from build123d import *

# Parameters (mm, degrees)
ESQUISSE2_W             = 33
ESQUISSE2_H             = 51
ENL_V_MAT_EXTRU_1_DEPTH = 41
ESQUISSE3_W             = 8
ESQUISSE3_H             = 12
ESQUISSE3_W_2           = 12
ESQUISSE3_H_2           = 8
ENL_V_MAT_EXTRU_3_DEPTH = 42
ESQUISSE4_W             = 23.524420498
ESQUISSE4_H             = 14.572913479
ENL_V_MAT_EXTRU_4_DEPTH = 269
ESQUISSE6_R             = 2.08560847
ENL_V_MAT_EXTRU_5_DEPTH = 10


with BuildPart() as part:
    # Esquisse1 → Révolution1 (revolve)
    with BuildSketch(Plane.XY, mode=Mode.PRIVATE) as r_volution1_sk:
        Polygon((0, 0), (-50, 0), (-35, 45), (0, 45), align=None)
    revolve(r_volution1_sk.sketch.rotate(Axis((0, 185.624886126, 0), (0, -1, 0)), 270), axis=Axis((0, 185.624886126, 0), (0, -1, 0)))

    # Esquisse2 → Enlèv. mat.-Extru.1 (cut)
    with BuildSketch(Plane(origin=(0, 45, 0), x_dir=(1, 0, 0), z_dir=(0, 1, 0))):
        Rectangle(ESQUISSE2_W, ESQUISSE2_H)
    extrude(amount=-ENL_V_MAT_EXTRU_1_DEPTH, mode=Mode.SUBTRACT)

    # Esquisse3 → Enlèv. mat.-Extru.3 (cut)
    with BuildSketch(Plane(origin=(0, 45, 0), x_dir=(1, 0, 0), z_dir=(0, 1, 0))):
        with Locations((0, 46)):
            Rectangle(ESQUISSE3_W, ESQUISSE3_H)
        with Locations((46, 0)):
            Rectangle(ESQUISSE3_W_2, ESQUISSE3_H_2)
        with Locations((0, -46)):
            Rectangle(ESQUISSE3_W, ESQUISSE3_H)
        with Locations((-46, 0)):
            Rectangle(ESQUISSE3_W_2, ESQUISSE3_H_2)
    extrude(amount=-ENL_V_MAT_EXTRU_3_DEPTH, mode=Mode.SUBTRACT)

    # Esquisse4 → Enlèv. mat.-Extru.4 (cut)
    with BuildSketch(Plane(origin=(0, 4, 0), x_dir=(1, 0, 0), z_dir=(0, 1, 0))):
        with Locations((-1.026102351, -0.627863405)):
            Rectangle(ESQUISSE4_W, ESQUISSE4_H)
    extrude(amount=-ENL_V_MAT_EXTRU_4_DEPTH, mode=Mode.SUBTRACT)

    # Esquisse6 → Enlèv. mat.-Extru.5 (cut)
    with BuildSketch(Plane(origin=(0, 3, 0), x_dir=(1, 0, 0), z_dir=(0, 1, 0))):
        with Locations(Location((0, 44.460655409, 0), (0, 0, 270))):
            Circle(ESQUISSE6_R)
    extrude(amount=-ENL_V_MAT_EXTRU_5_DEPTH, mode=Mode.SUBTRACT)


solid = part.part
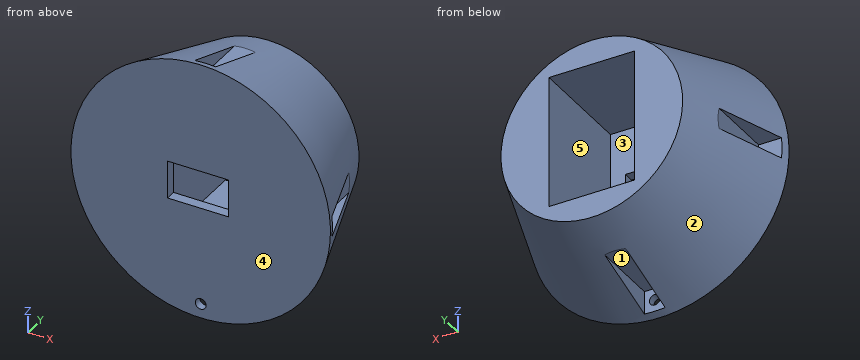
Read the model definition and answer for the solid it produces. Units are mm, in the model's axes. Face numbers are marked on the shaded views. A direction names the side the tool comes from. Give positions to 0.01 mm unless a question says otherwise; leave off trailing zeros. Loops run counter-clockwise (first coordinate to the right, second up) from the corner with the lowest first, then second, coordinate; pieces in that order, holes last. Notation, with made-up numbers: M 22,39.5 L 36,39.5 A19 ccw 36,69.5 Z; hole C -33.5,-34 d6. An arc over 180 degrees is marked long. Write each question's results on one line, items separated by ' | '.
1. Section A-A on z = 0 is taken. Give the vertices of the cut face in (x, y), plus the area to 3 significant figures.
Values:
outline: M -50,0 L -12.79,0 L -12.79,4 L -16.5,4 L -16.5,45 L -35,45 L -40,30 L -40,3 L -49,3 Z; M 10.74,0 L 50,0 L 49,3 L 40,3 L 40,30 L 35,45 L 16.5,45 L 16.5,4 L 10.74,4 Z | area: 2,130 mm^2
2. A tool of negligible diameter and unlimited length cuts with its end or side. For the marked faces 4 and 5, from which of +Z, -Z, +X, -X, +Y, -Y can it reach the whole face along a straight path? Write none if from no direction.
Values:
face 4: +Z, -Z, +X, -X, -Y | face 5: +Y
3. Section B-B on y = 37.5 is taken. Give the vertices of the cut face in (x, z).
Values:
outline: C 0,0 d75; hole M -16.5,-25.5 L 16.5,-25.5 L 16.5,25.5 L -16.5,25.5 Z
4. The mould has two halves that part along Z. Classify the marked faces 1, 2 and 3: pulls with the +Z half, pulls with the -Z half, needs draft (parallel to the pull), parting line crosses it, or undercut.
Values:
face 1: pulls with the -Z half | face 2: parting line crosses it | face 3: undercut
5. Straight lines are drawn through the part: line 1 (Z direction, x = 3.5, y = 29); line 2 (X direction, y = 17, z = -3); line 3 (Y direction, x = 14.5, z = 8.5). For each, find the intervals that lie inside material, in ascending order. Write a range as [from, to].
Values:
line 1: z = [-40, -25.5], [25.5, 40] | line 2: x = [-40, -16.5], [16.5, 40] | line 3: y = [0, 4]
6. Section C-C on x = 0 is taken. Give the vertices of the cut face in (y, z), plus the area to 3 significant figures.
Values:
outline: M 0,-50 L 3,-49 L 3,-46.55 L 0,-46.55 Z; M 0,-42.38 L 3,-42.38 L 3,-40 L 30,-40 L 45,-35 L 45,-25.5 L 4,-25.5 L 4,-6.66 L 0,-6.66 Z; M 0,7.91 L 4,7.91 L 4,25.5 L 45,25.5 L 45,35 L 30,40 L 3,40 L 3,49 L 0,50 Z | area: 1,420 mm^2
7. Section D-D on y = 12.5 is taken. Give the vertices of the cut face in (x, z).
Values:
outline: M -45.66,-4 A45.83 ccw -4,-45.66 L -4,-40 L 4,-40 L 4,-45.66 A45.83 ccw 45.66,-4 L 40,-4 L 40,4 L 45.66,4 A45.83 ccw 4,45.66 L 4,40 L -4,40 L -4,45.66 A45.83 ccw -45.66,4 L -40,4 L -40,-4 Z; hole M -16.5,-25.5 L 16.5,-25.5 L 16.5,25.5 L -16.5,25.5 Z
8. Given pin 1 (4 mm diameter, centred on y = 29, z = 10.5, fed in from -X); pin 2 (1.2 mm diameter, centred on y = 1, z = 0.5, fed in from +X); pin 3 (2 mm diameter, centred on x = 13.5, y = 7, fed in from +Z), each flat-ended and moving along its own axis, determine where each tip first touches the part or whether it passes through.
Values:
pin 1: stops at x = -39.8 | pin 2: stops at x = 49.86 | pin 3: stops at z = 46.17
